Source: CAD feature listing. Evaluate the final solid. Frame: model axes, mm. Round coordinates to 2 decimals unless told otherwise and drop trailing zeros. Answer as CSV lines item,"result". Start each with the question number.
(1) Contact query for a flat-ended pin moving along its axis: P1, Ø1.8, axis at x = 40, y = 40, coming from the -Z side. Output: stop coordinate, or through.
(2) Line query: line 1 along Y through (x, z) = (10, 1.75); line 2 along X through (y, z) = (11, 2.55); line 3 along Y through (x, z) = (39, 2.6). Output: solid intervals per line, ascending. Write a range as from..to.
(3) Pull-direction query (Z, two-part tool) for faces 1 (the flat face through (108, 25, 3)), 2 (the flat face through (108, 25, 0)); classes: +Z half, -Z half, draft (parallel to the pull), parting line (faces both ways), or undercut.
Autodesk Inventor part; units mm, degrees
ref_plane "YZ Plane" through (0, 0, 0) normal (1, 0, 0) x (0, 1, 0)
ref_plane "XZ Plane" through (0, 0, 0) normal (0, 1, 0) x (-1, 0, 0)
ref_plane "XY Plane" through (0, 0, 0) normal (0, 0, 1) x (1, 0, 0)
sketch "Sketch1" plane through (0, 0, 0) normal (0, 0, 1) x (1, 0, 0)
  circle A0 centre (6.0619, 42.5) radius 1.5
  circle A1 centre (6.0619, 7.5) radius 1.5
  circle A2 centre (28.8092, 42.5) radius 1.5
  circle A3 centre (28.8092, 7.5) radius 1.5
  line L0 (34.8712, 0) -> (0, 0)
  line L1 (34.8712, 0) -> (34.8712, 50)
  line L2 (0, 50) -> (34.8712, 50)
  line L3 (0, 0) -> (0, 50)
  line L4 (0, 0) -> (220, 0)
  line L5 (220, 0) -> (220, 50)
  line L6 (220, 50) -> (0, 50)
  line L7 (0, 50) -> (0, 0)
  point P0 (19, 50)
  point P1 (19, 0)
  dimension "d0" = 220
  dimension "d1" = 50
extrude "Extrusion1" add sketch "Sketch1" along normal blind 3 contours A0 | A1 | A2 | A3 | L0 L3 L2 L1 | L1 L6 L5 L4
sketch "Sketch2" plane through (0, 0, 0) normal (0, 0, -1) x (-1, 0, 0)
  arc A0 (-300, 50) -> (-310, 40) centre (-300, 40) ccw
  line L0 (-310, 40) -> (-310, 10)
  arc A1 (-310, 10) -> (-300, 0) centre (-300, 10) ccw
  line L1 (-300, 0) -> (-170, 0)
  line L2 (-170, 0) -> (-170, 50)
  line L3 (-170, 50) -> (-300, 50)
  circle A2 centre (-250.5156, 19.2053) radius 1.75
  circle A3 centre (-250.7947, 30.5156) radius 1.75
  circle A4 centre (-239.2053, 19.4844) radius 1.75
  circle A5 centre (-239.4844, 30.7947) radius 1.75
  circle A6 centre (-263.75, 25) radius 2.6
  circle A7 centre (-280, 25) radius 5
  circle A8 centre (-296.25, 25) radius 2.6
  circle A9 centre (-245, 25) radius 5.5
  circle A10 centre (-210, 40) radius 1.5
  circle A11 centre (-210, 10) radius 1.5
  circle A12 centre (-180, 40) radius 1.5
  circle A13 centre (-180, 10) radius 1.5
  line L4 (-50, 0) -> (55, 0)
  arc A14 (55, 0) -> (65, 10) centre (55, 10) ccw
  line L5 (65, 10) -> (65, 40)
  arc A15 (65, 40) -> (55, 50) centre (55, 40) ccw
  line L6 (55, 50) -> (-50, 50)
  line L7 (-50, 50) -> (-50, 0)
  circle A16 centre (-40, 40) radius 1.5
  circle A17 centre (-40, 10) radius 1.5
  circle A18 centre (36, 25) radius 5
  circle A19 centre (19.75, 25) radius 2.6
  circle A20 centre (52.25, 25) radius 2.6
  circle A21 centre (-10, 40) radius 1.5
  circle A22 centre (-10, 10) radius 1.5
  point P0 (0, 0)
extrude "Extrusion2" cut sketch "Sketch2" against normal through all contours A10 | A11 | A12 | A13 | A16 | A17
ref_plane "Work Plane1" through (110, 0, 0) normal (1, 0, 0) x (0, 0, -1)
mirror "Mirror1" about plane through (110, 0, 0) normal (1, 0, 0) of "Extrusion2"
properties part number "arm1" material "Polycarbonate, Clear"
Answer block:
1,P1,"through"
2,line 1,"0..8.5, 11.5..38.5, 41.5..50"
2,line 2,"0..8.88, 11.12..38.88, 41.12..178.88, 181.12..208.88, 211.12..220"
2,line 3,"0..8.88, 11.12..38.88, 41.12..50"
3,face 1,"+Z half"
3,face 2,"-Z half"
